Autodesk Fusion 360 part; units mm, degrees
sketch "Sketch1" plane through (0, 0, 0) normal (0, 1, 0) x (1, 0, 0)
  line L0 (0, 0) -> (-68, 0)
  line L1 (-68, 0) -> (-68, -24)
  line L2 (-68, -24) -> (0, -24)
  line L3 (0, -24) -> (0, 0)
extrude "Extrude1" add sketch "Sketch1" along normal blind 2
sketch "Sketch2" plane through (0, 0, 0) normal (0, 1, 0) x (1, 0, 0)
  line L0 (-66, -22) -> (0, -22)
  line L1 (0, -22) -> (0, -20)
  line L2 (0, -20) -> (-66, -20)
  line L3 (-66, -20) -> (-66, -22)
extrude "Extrude2" add sketch "Sketch2" against normal blind 2
sketch "Sketch3" plane through (0, 0, 0) normal (0, 1, 0) x (1, 0, 0)
  line L0 (-66, -20) -> (-64, -20)
  line L1 (-64, -20) -> (-64, -2)
  line L2 (-64, -2) -> (-66, -2)
  line L3 (-66, -2) -> (-66, -20)
extrude "Extrude3" add sketch "Sketch3" against normal blind 2
sketch "Sketch4" plane through (0, 0, 0) normal (0, 1, 0) x (1, 0, 0)
  line L0 (-64, -4) -> (0, -4)
  line L1 (0, -4) -> (0, -2)
  line L2 (0, -2) -> (-64, -2)
  line L3 (-64, -2) -> (-64, -4)
extrude "Extrude4" add sketch "Sketch4" against normal blind 2
sketch "Sketch5" plane through (0, 0, 0) normal (0, 1, 0) x (1, 0, 0)
  line L0 (-10, -22) -> (0, -22)
  line L1 (0, -22) -> (0, -20)
  line L2 (0, -20) -> (-10, -20)
  line L3 (-10, -20) -> (-10, -22)
extrude "Extrude5" add sketch "Sketch5" against normal blind 10
extrude "Extrude6" add 1 faces at (-6.6667, -10, 20.6667) along direction (0, -1, 0) blind 5
sketch "Sketch6" plane through (0, 0, 0) normal (0, 1, 0) x (1, 0, 0)
  line L0 (-10, -4) -> (0, -4)
  line L1 (0, -4) -> (0, -2)
  line L2 (0, -2) -> (-10, -2)
  line L3 (-10, -2) -> (-10, -4)
extrude "Extrude7" add sketch "Sketch6" against normal blind 15
Could you check a few things on this model? Use its own coordinates, in mm. A direction names the side the tool comes from. Give positions to 0.01 mm unless a question says otherwise; leave off trailing zeros. Write each loop counter-clockwise with the first axis right and the second up, starting at its lowest first coordinate (ties: lowest second). Pieces come first, ordered by that corner, then holes. Notation, with made-up numbers: (-17.5, 40) - (21.5, 40) arc R17 cw to (21.5, 58) - close; hole circle Ø10 at (29.25, 31). An arc over 180 degrees is marked (long way). Use CSV: the item, a comma, the result in double quotes. Start each with the question number.
Item 1: I want a section at B-B, the plane y = -6.25. Please give me the cut outline in (x, z).
Item 2: For faces 4 (the face through (-66, -1, 12)), 5 (the face through (-21, -1, 22)), 6 (the face through (-32, 0, 12)), which set-ups out of +Z, -Z, +X, -X, +Y, -Y let a thin tool reach every point of the face, with its end or its side?
Item 3: I'm going to push flat-ended pins straight in: pin 1 (4.5 mm diameter, centred on x = -29.5, y = -4, fed in from +Z); pin 2 (0.6 mm diameter, centred on y = -7.5, z = 21, fed in from -X); pin 3 (10 mm diameter, centred on x = -28.5, z = 7.5, fed in from -Y). Where does each tip first touch, or does it pass through?
Item 4: If we mould it in two halves opening along Z, with no side actions, what happens to faces 1 (the face through (-21, -1, 2)), 2 (the face through (-20, -1, 4)), 3 (the face through (-34, 1, 24))? For each: pulls with the +Z half, pulls with the -Z half, needs draft (parallel to the pull), parting line crosses it, or undercut.
Item 5: I want a section at C-C, the plane x = -8. Please give me the cut outline in (y, z).
Item 6: If I drill on line 1 along Z through (x, y) = (-49.5, -0.25); line 2 along X through (y, z) = (-1.25, 16.5); line 3 along Y through (x, z) = (-4.5, 15.5), over which ranges is the centre line in solid material (lowest first)?
Item 7: I want a section at D-D, the plane x = -40.5. Please give me the cut outline in (y, z), then the cut area to 3 significant figures.
Item 8: I want a section at A-A, the plane z = 8.75. Please give me the cut outline in (x, y), then the cut area to 3 significant figures.
Findings:
1,outline,"(-10, 2) - (0, 2) - (0, 4) - (-10, 4) - close; (-10, 20) - (0, 20) - (0, 22) - (-10, 22) - close"
2,face 4,"+Z, -Z, -X, -Y"
2,face 5,"+Z, +X, -X, -Y"
2,face 6,"+X, -Y"
3,pin 1,"stops at z = 22"
3,pin 2,"stops at x = -10"
3,pin 3,"stops at y = -2"
4,face 1,"pulls with the -Z half"
4,face 2,"undercut"
4,face 3,"pulls with the +Z half"
5,outline,"(-15, 2) - (0, 2) - (0, 0) - (2, 0) - (2, 24) - (0, 24) - (0, 22) - (-15, 22) - (-15, 20) - (0, 20) - (0, 4) - (-15, 4) - close"
6,line 1,"z = 2 to 4, 20 to 22"
6,line 2,"x = -66 to -64"
6,line 3,"y = 0 to 2"
7,outline,"(-2, 2) - (0, 2) - (0, 0) - (2, 0) - (2, 24) - (0, 24) - (0, 22) - (-2, 22) - (-2, 20) - (0, 20) - (0, 4) - (-2, 4) - close"
7,area,"56.0 mm2"
8,outline,"(-68, 0) - (-66, 0) - (-66, -2) - (-64, -2) - (-64, 0) - (0, 0) - (0, 2) - (-68, 2) - close"
8,area,"140 mm2"
